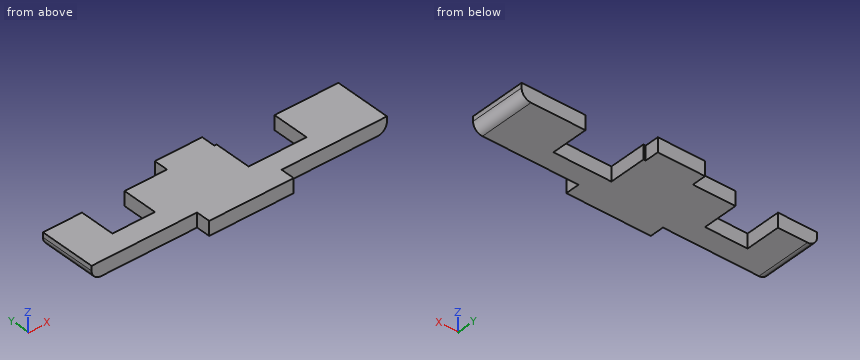
from build123d import *

# Parameters (mm, degrees)
SKETCH1_W           = 62.46
SKETCH1_H           = 18
BOSS_EXTRUDE1_DEPTH = 3
SKETCH2_W           = 22.295
SKETCH2_H           = 3
CUT_EXTRUDE1_DEPTH  = 3
SKETCH3_W           = 12.25
SKETCH3_H           = 10.9
SKETCH3_W_2         = 9
SKETCH3_H_2         = 10.5
CUT_EXTRUDE2_DEPTH  = 3
SKETCH5_W           = 26.23
SKETCH5_H           = 3
CUT_EXTRUDE3_DEPTH  = 3
FILLET1_R           = 2
FILLET2_R           = 2


with BuildPart() as part:
    # Sketch1 → Boss-Extrude1 (new body)
    with BuildSketch(Plane.XY):
        Rectangle(SKETCH1_W, SKETCH1_H)
    extrude(amount=BOSS_EXTRUDE1_DEPTH)

    # Sketch2 → Cut-Extrude1 (cut)
    with BuildSketch(Plane.XY.offset(3)):
        with Locations((20.0825, -7.5)):
            Rectangle(SKETCH2_W, SKETCH2_H)
        with Locations((-20.0825, -7.5)):
            Rectangle(SKETCH2_W, SKETCH2_H)
    extrude(amount=-CUT_EXTRUDE1_DEPTH, mode=Mode.SUBTRACT)

    # Sketch3 → Cut-Extrude2 (cut)
    with BuildSketch(Plane.XY.offset(3)):
        with Locations((11.605, 3.55)):
            Rectangle(SKETCH3_W, SKETCH3_H)
        with Locations((-18.48, 3.75)):
            Rectangle(SKETCH3_W_2, SKETCH3_H_2)
    extrude(amount=-CUT_EXTRUDE2_DEPTH, mode=Mode.SUBTRACT)

    # Sketch5 → Cut-Extrude3 (cut)
    with BuildSketch(Plane(origin=(0, 0, 0), x_dir=(-1, 0, 0), z_dir=(0, 0, -1))):
        with Locations((18.115, 7.5)):
            Rectangle(SKETCH5_W, SKETCH5_H)
        with Locations((-18.115, 7.5)):
            Rectangle(SKETCH5_W, SKETCH5_H)
    extrude(amount=-CUT_EXTRUDE3_DEPTH, mode=Mode.SUBTRACT)

    # Fillet1
    fillet1_edges = [part.edges().sort_by_distance(p)[0] for p in [
        (-31.23, 0, 0),
    ]]
    fillet(fillet1_edges, radius=FILLET1_R)

    # Fillet2
    fillet2_edges = [part.edges().sort_by_distance(p)[0] for p in [
        (31.23, 0, 0),
    ]]
    fillet(fillet2_edges, radius=FILLET2_R)


solid = part.part
For this review, take the finished solid that the model builds, in its own axes (mm). Round coordinates to 2 decimals unless told otherwise and drop trailing zeros. Write each loop counter-clockwise with the first axis right and the second up, starting at its lowest first coordinate (ties: lowest second). Pieces come first, ordered by that corner, then holes. Notation, with made-up numbers: (37.25, 8.25) - (68.25, 8.25) arc R19 cw to (68.25, 29.25) - close; hole circle Ø3 at (39, 86.25). An arc over 180 degrees is marked (long way). Use a Markdown table: item, result.
Q1. Clearance check with flat-ended pins moving along their axes: pin 1 (0.9 mm diameter, centred on x = 23, z = 1, fed in from -Y); pin 2 (1.5 mm diameter, centred on x = -23.5, z = 0.5, fed in from +Y); pin 3 (1 mm diameter, centred on x = 10.5, z = 1, fed in from +Y). State where each tip first meets the part, or that it passes through.
Derived:
| item | result |
|---|---|
| pin 1 | stops at y = -6 |
| pin 2 | stops at y = 6 |
| pin 3 | stops at y = -1.9 |
Q2. We need section A-A (y = 0.25). Give the boundary of the cut face in (x, z), plus the area to 3 significant figures.
Derived:
| item | result |
|---|---|
| outline | (-31.23, 2) arc R2 ccw to (-29.23, 0) - (-22.98, 0) - (-22.98, 3) - (-31.23, 3) - close; (-13.98, 0) - (5.48, 0) - (5.48, 3) - (-13.98, 3) - close; (17.73, 0) - (29.23, 0) arc R2 ccw to (31.23, 2) - (31.23, 3) - (17.73, 3) - close |
| area | 122 mm2 |
Q3. We need section D-D (x = -6.5). Give the boundary of the cut face in (y, z).
Derived:
| item | result |
|---|---|
| outline | (-9, 0) - (6, 0) - (6, 3) - (-9, 3) - close |
Q4. We need section C-C (x = 25). Give the boundary of the cut face in (y, z).
Derived:
| item | result |
|---|---|
| outline | (-6, 0) - (6, 0) - (6, 3) - (-6, 3) - close |
Q5. Wall thickness on line 1 along X through (y, z) = (0.25, 1.85); line 2 along X through (y, z) = (3, 1.25); line 3 along Y through (x, z) = (21, 0.5): over which ranges is each line inside the solid? List them lowest first.
Derived:
| item | result |
|---|---|
| line 1 | x = -31.22 to -22.98, -13.98 to 5.48, 17.73 to 31.22 |
| line 2 | x = -31.08 to -22.98, -13.98 to 5.48, 17.73 to 31.08 |
| line 3 | y = -6 to 6 |
Q6. We need section B-B (z = 0.85). Give the boundary of the cut face in (x, y) (3 decimals).
Derived:
| item | result |
|---|---|
| outline | (-30.866, -6) - (-8.935, -6) - (-8.935, -9) - (8.935, -9) - (8.935, -6) - (30.866, -6) - (30.866, 6) - (17.73, 6) - (17.73, -1.9) - (5.48, -1.9) - (5.48, 6) - (5, 6) - (5, 9) - (-5, 9) - (-5, 6) - (-13.98, 6) - (-13.98, -1.5) - (-22.98, -1.5) - (-22.98, 6) - (-30.866, 6) - close |
